from build123d import *

# Parameters (mm, degrees)
SKETCH001_W  = 470
SKETCH001_H  = 8
PAD001_DEPTH = 4
CHAMFER_SIZE = 7.99
FILLET_R     = 7.99


with BuildPart() as part:
    # Sketch001 → Pad001 (new body, symmetric)
    with BuildSketch(Plane.XZ):
        Rectangle(SKETCH001_W, SKETCH001_H)
    extrude(amount=PAD001_DEPTH, both=True)

    # Chamfer
    chamfer_edges = [part.edges().sort_by_distance(p)[0] for p in [
        (235, 0, 4),
        (-235, 0, 4),
    ]]
    chamfer(chamfer_edges, length=CHAMFER_SIZE)

    # Fillet
    fillet_edges = [part.edges().sort_by_distance(p)[0] for p in [
        (0, 4, 4),
    ]]
    fillet(fillet_edges, radius=FILLET_R)


solid = part.part
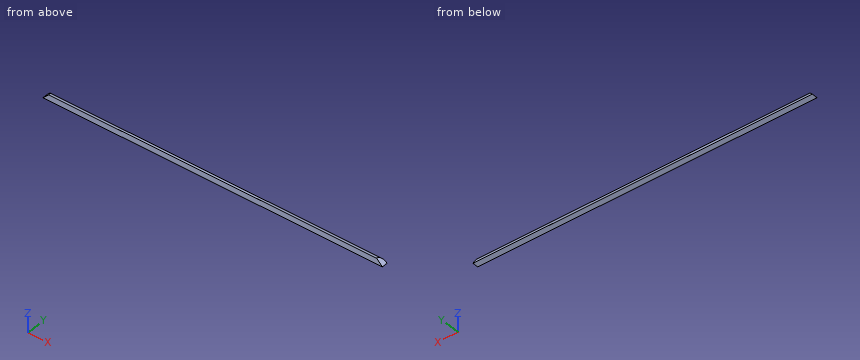
Verification items for the finished model (mm, model axes). Coordinates: 2 decimals unless noted, no trailing zeros. Loops run counter-clockwise (first coordinate to the right, second up) from the corner with the lowest first, then second, coordinate; pieces in that order, holes last. Notation, with made-up numbers: (79, -29) -> (93, -29) arc R16 cw to (93, -13) -> close; hole circle Ø9 at (24, -40). An arc over 180 degrees is marked (long way). Answer as a JSON object with one key per item and string values. Group by question number.
Item 1: Sectioned sample at C-C on z = -0.5. Record the boundary of the cut face in (x, y).
Item 2: Scan lines: probe 1 along Y at (x, z) = (-132, -3.25); probe 2 along Y at (x, z) = (168.5, -3); probe 3 along Z at (x, y) = (54, -1). Record each from-to range of solid material in increasing order.
Item 3: Depth check by flat-ended pin: pin 1 (1 mm diameter, centred on y = -2, z = -0.5, fed in from -X); pin 2 (4 mm diameter, centred on y = 1, z = 2.5, fed in from -X); pin 3 (1 mm diameter, centred on y = 0.5, z = 2, fed in from +X). Enter the tip coordinate at first touch or a pass-through.
Evaluation:
{
 "1": {"outline": "(-231.51, -4) -> (231.51, -4) -> (231.51, 3.2) -> (-231.51, 3.2) -> close"},
 "2": {"probe 1": "y = -4 to 3.97", "probe 2": "y = -4 to 3.94", "probe 3": "z = -4 to 3.42"},
 "3": {"pin 1": "stops at x = -232.01", "pin 2": "stops at x = -230.51", "pin 3": "stops at x = 229.51"}
}
